Design review of the part built by this model. Coordinates are the model's own, in mm. A direction names the side the tool comes from. Give positions to 0.01 mm unless a question says otherwise; leave off trailing zeros. Write each loop counter-clockwise with the first axis right and the second up, starting at its lowest first coordinate (ties: lowest second). Pieces come first, ordered by that corner, then holes. Notation, with made-up numbers: (54.5, 1) -> (98.5, 1) arc R27 cw to (98.5, 40) -> close; hole circle Ø11 at (55, -28.75). An arc over 180 degrees is marked (long way). Use CSV: the item, a comma, the result in double quotes.
```python
from build123d import *

# Parameters (mm, degrees)
F0_R     = 7
F1_DEPTH = 21.5
F2_R     = 5


with BuildPart() as f1:
    # F0 (on Front) → F1 (new body, symmetric)
    with BuildSketch(Plane.XZ):
        with BuildLine():
            Line((-9.187381455, 19.4473182438), (-26.5, 22.5))
            Line((-26.5, 22.5), (-33.5, 22.5))
            Line((-33.5, 22.5), (-40.5, 15.5))
            Line((-40.5, 15.5), (-40.5, -2.5))
            Line((-40.5, -2.5), (-33.5, -9.5))
            Line((-33.5, -9.5), (-0.733982586, -9.5))
            ThreePointArc((-0.733982586, -9.5), (1.3935612661, -18.5714631594), (6.2880673968, -26.5))
            Line((6.2880673968, -26.5), (11.5, -26.5))
            Line((11.5, -26.5), (40.5, 6.5))
            Line((40.5, 6.5), (40.5, 25.5))
            Line((40.5, 25.5), (35.5, 30.5))
            Line((35.5, 30.5), (11.5, 30.5))
            ThreePointArc((11.5, 30.5), (3.0653504529, 21.400493443), (-9.187381455, 19.4473182438))
        make_face()
        with Locations((-26.5, 4.5)):
            Circle(F0_R, mode=Mode.SUBTRACT)
    extrude(amount=F1_DEPTH, both=True)

    # F2
    f2_edges = [f1.edges().sort_by_distance(p)[0] for p in [
        (-0.733983, 0, -9.5),
    ]]
    fillet(f2_edges, radius=F2_R)


solid = f1.part
```
(1) For line 1 along Z through (x, y) = (-26.5, 1.5); line 2 along X through (y, z) = (10.5, 5.5); line 3 along Z through (x, y) = (-30, -17), list the stretches that pass through material, from the lowest coordinate up. Write a range as [from, to].
Established:
line 1,"z = [-9.5, -2.5], [11.5, 22.5]"
line 2,"x = [-40.5, -33.43], [-19.57, 39.62]"
line 3,"z = [-9.5, -1.56], [10.56, 22.5]"
(2) Clearance check with flat-ended pins moving along their axes: pin 1 (10 mm diameter, centred on x = 4.5, y = 11.5, fed in from +Z); pin 2 (2 mm diameter, centred on x = -30.5, y = 8.5, fed in from +Z); pin 3 (2 mm diameter, centred on x = -18.5, y = -11.5, fed in from -Z); pin 4 (5 mm diameter, centred on x = 1.5, z = 24.5, fed in from +Y). State where each tip first meets the part, or that it passes through.
Established:
pin 1,"stops at z = 27.01"
pin 2,"stops at z = 22.5"
pin 3,"stops at z = -9.5"
pin 4,"passes through"
(3) Take a section at A-A (y = 5.5). Write out the cut boundary in (x, z), then the cut area to 3 significant figures.
Established:
outline,"(-40.5, -2.5) -> (-33.5, -9.5) -> (-5.07, -9.5) arc R5 cw to (-0.18, -13.47) arc R29 ccw to (6.29, -26.5) -> (11.5, -26.5) -> (40.5, 6.5) -> (40.5, 25.5) -> (35.5, 30.5) -> (11.5, 30.5) arc R19 cw to (-9.19, 19.45) -> (-26.5, 22.5) -> (-33.5, 22.5) -> (-40.5, 15.5) -> close; hole circle Ø14 at (-26.5, 4.5)"
area,"2,750 mm2"
(4) Tool access review of faces 5 (the face through (-19, 0, -9.5)), 6 (the face through (-30, 0, 22.5)), 7 (the face through (-18, 0, 21)): name each direction out of +Z, -Z, +X, -X, +Y, -Y from which nothing blocks a thin tool from reaching the whole face with its end or side.
Established:
face 5,"-Z, -X, +Y, -Y"
face 6,"+Z, -X, +Y, -Y"
face 7,"+Z, +Y, -Y"
(5) Take a section at B-B (z = -1.5). Write out the cut boundary in (x, y).
Established:
outline,"(-40.5, -21.5) -> (-30.11, -21.5) -> (-30.11, 21.5) -> (-40.5, 21.5) -> close; (-22.89, -21.5) -> (33.47, -21.5) -> (33.47, 21.5) -> (-22.89, 21.5) -> close"
(6) Mouldability with a two-part tool opening along X and no side actions: class faces 1 (the face through (3.221, -0.301, 21.485)), 2 (the face through (24, 0, 30.5)), 3 (the face through (-19.823, 0.301, 6.603)), 4 (the face through (2.18, -0.3, -20.31)) as +X half, -X half, draft (parallel to the pull), parting line (faces both ways), or undercut.
Established:
face 1,"undercut"
face 2,"draft"
face 3,"undercut"
face 4,"-X half"
(7) Take a section at D-D (x = 24). Write out the cut boundary in (y, z).
Established:
outline,"(-21.5, -12.28) -> (21.5, -12.28) -> (21.5, 30.5) -> (-21.5, 30.5) -> close"
(8) Take a section at C-C (x = -21). Write out the cut boundary in (y, z), then the cut area to 3 significant figures.
Established:
outline,"(-21.5, -9.5) -> (21.5, -9.5) -> (21.5, 0.17) -> (-21.5, 0.17) -> close; (-21.5, 8.83) -> (21.5, 8.83) -> (21.5, 21.53) -> (-21.5, 21.53) -> close"
area,"962 mm2"
